Model file for the job. Use its own axes, mm. Round coordinates to 2 decimals unless told otherwise and drop trailing zeros. Loops run counter-clockwise (first coordinate to the right, second up) from the corner with the lowest first, then second, coordinate; pieces in that order, holes last. Notation, with made-up numbers: (33.5, 89) - (47.5, 89) arc R30 ccw to (47.5, 115) - close; hole circle Ø2 at (57, 68). An arc over 180 degrees is marked (long way). Use one line per item in the form item = value.
Autodesk Inventor part; units mm, degrees
ref_plane "YZ Plane" through (0, 0, 0) normal (1, 0, 0) x (0, 1, 0)
ref_plane "XZ Plane" through (0, 0, 0) normal (0, 1, 0) x (-1, 0, 0)
ref_plane "XY Plane" through (0, 0, 0) normal (0, 0, 1) x (1, 0, 0)
sketch "Skizze1" plane through (0, 0, 0) normal (0, 0, 1) x (1, 0, 0)
  line L0 (-182, -120) -> (182, -120)
  line L1 (182, -120) -> (182, 120)
  line L2 (182, 120) -> (-182, 120)
  line L3 (-182, 120) -> (-182, -120)
  line L4 (-182, -120) -> (182, 120) construction
  line L5 (182, -120) -> (-182, 120) construction
  circle A0 centre (0, 0) radius 36.5
  line L6 (-140, -90) -> (140, -90)
  line L7 (140, -90) -> (140, 90)
  line L8 (140, 90) -> (-140, 90)
  line L9 (-140, 90) -> (-140, -90)
  line L10 (-140, -90) -> (140, 90) construction
  line L11 (140, -90) -> (-140, 90) construction
  circle A1 centre (-140, 90) radius 3.25
  circle A2 centre (140, 90) radius 3.25
  circle A3 centre (140, -90) radius 3.25
  circle A4 centre (-140, -90) radius 3.25
  point P0 (0, 0)
  point P1 (0, 0)
  point P2 (0, 0)
  dimension "d0" = 364
  dimension "d1" = 240
  dimension "d5" = 73
  dimension "d6" = 280
  dimension "d7" = 180
  dimension "d8" = 6.5
extrude "Extrusion1" add sketch "Skizze1" along normal blind 18 contours L3 L2 L1 L0 | L9 A4 L6 | L6 A4 L9 | A4 L9 A1 L8 A2 L7 A3 L6 | A3 L7 L6 | L6 L7 A3 | A1 L8 L9 | L9 L8 A1 | A2 L8 L7 | L7 L8 A2
extrude "Extrusion2" cut sketch "Skizze1" along normal through all contours L9 A4 L6 | L6 A4 L9 | A3 L7 L6 | L6 L7 A3 | A1 L8 L9 | L9 L8 A1 | A2 L8 L7 | L7 L8 A2
equation "\"d0\" = case_width - 2 * case_thickness"
equation "\"d1\" = inner_depth - inner_thickness"
equation "\"d2\" = case_thickness"
equation "\"kg_thickness\" = 4.9"
equation "\"ht_thickness\" = 1.9"
equation "\"case_thickness\" = 18"
equation "\"inner_thickness\" = 15"
equation "\"gap_fit\" = 0.1"
equation "\"gap_slide\" = 0.2"
equation "\"gap_air\" = 1"
equation "\"bore_diameter\" = 73"
equation "\"mdf_thickness\" = 6"
equation "\"tape_width\" = 15"
equation "\"tape_thickness\" = 3"
equation "\"inner_depth\" = 255"
properties part number "Korpus_Einbau_Basis"
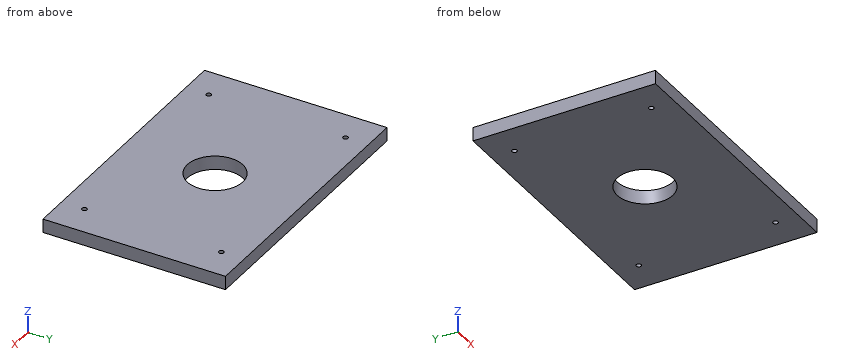
1. Flat gauge pin, fed straight in: pin 1 (8.5 mm diameter, centred on x = -140, y = 90, fed in from +Z). Where does the tip first touch, or does it go through?
Geometry check:
pin_1 = 18
2. Cut at B-B, the plane z = 13.25. Give the cut face in (x, y).
Geometry check:
outline = (-182, -120) - (182, -120) - (182, 120) - (-182, 120) - close; hole circle Ø6.5 at (-140, -90); hole circle Ø6.5 at (-140, 90); hole circle Ø73 at (0, 0); hole circle Ø6.5 at (140, -90); hole circle Ø6.5 at (140, 90)
3. Cut at A-A, the plane x = 0. Give the cut face in (y, z), plus the area to 3 significant figures.
Geometry check:
outline = (-120, 0) - (-36.5, 0) - (-36.5, 18) - (-120, 18) - close; (36.5, 0) - (120, 0) - (120, 18) - (36.5, 18) - close
area = 3,010 mm^2
4. Wall check: probe 1 along Y at (x, z) = (140, 5.75); probe 2 along X at (y, z) = (90, 4); probe 3 along Y at (x, z) = (0, 11.5). Give the ranges that are in metal, low to high.
Geometry check:
probe_1 = -120 to -93.25, -86.75 to 86.75, 93.25 to 120
probe_2 = -182 to -143.25, -136.75 to 136.75, 143.25 to 182
probe_3 = -120 to -36.5, 36.5 to 120
